```python
from build123d import *

# Parameters (mm, degrees)
SKETCH1_R               = 65
BULK_EXTRUDE_DEPTH      = 3
SKETCH2_R               = 40.5
SKETCH2_R_2             = 37.5
BEARING_RING_DEPTH      = 6
BEARING_START           = -1
SKETCH4_R               = 37.5
BEARING_CUT_DEPTH       = 1
SKETCH5_R               = 22
WIRE_PASSTHRU_CUT_DEPTH = 143.214667503


with BuildPart() as part:
    # Sketch1 → BULK EXTRUDE (new body)
    with BuildSketch(Plane(origin=(72, 0, 0), x_dir=(0, 0, -1), z_dir=(1, 0, 0))):
        with Locations((50, -18.372727273)):
            Circle(SKETCH1_R)
    extrude(amount=BULK_EXTRUDE_DEPTH)

    # Sketch2 → BEARING RING (add)
    with BuildSketch(Plane(origin=(75, 0, 0), x_dir=(0, 0, -1), z_dir=(1, 0, 0))):
        with Locations((50, -18.372727273)):
            Circle(SKETCH2_R)
        with Locations((50, -18.372727273)):
            Circle(SKETCH2_R_2, mode=Mode.SUBTRACT)
    extrude(amount=BEARING_RING_DEPTH)

    # Sketch4 → BEARING CUT (cut)
    with BuildSketch(Plane(origin=(75, 0, 0), x_dir=(0, 0, -1), z_dir=(1, 0, 0)).offset(BEARING_START)):
        with Locations((50, -18.372727273)):
            Circle(SKETCH4_R)
    extrude(amount=BEARING_CUT_DEPTH, mode=Mode.SUBTRACT)

    # Sketch5 → WIRE PASSTHRU CUT (cut, through all)
    with BuildSketch(Plane(origin=(74, 0, 0), x_dir=(0, 0, -1), z_dir=(1, 0, 0))):
        with Locations((50, -18.372727273)):
            Circle(SKETCH5_R)
    extrude(amount=-WIRE_PASSTHRU_CUT_DEPTH, mode=Mode.SUBTRACT)


solid = part.part
```
Geometry check sheet. Reference: the model listing, model coordinates, mm. A direction names the side the tool comes from. Give positions to 0.01 mm unless a question says otherwise; leave off trailing zeros. Loops run counter-clockwise (first coordinate to the right, second up) from the corner with the lowest first, then second, coordinate; pieces in that order, holes last. Notation, with made-up numbers: M 28.25,89 L 59.25,89 A35 ccw 59.25,128 Z; hole C 15.25,11.25 d10. An arc over 180 degrees is marked long. Write item = value, one per line.
(1) Sectioned sample at A-A, the plane z = -50. Record the cut outline in (x, y), plus the area to 3 significant figures.
Answer below:
outline = M 72,-83.37 L 75,-83.37 L 75,-58.87 L 81,-58.87 L 81,-55.87 L 74,-55.87 L 74,-40.37 L 72,-40.37 Z; M 72,3.63 L 74,3.63 L 74,19.13 L 81,19.13 L 81,22.13 L 75,22.13 L 75,46.63 L 72,46.63 Z
area = 263 mm2
(2) Sectioned sample at D-D, the plane y = -47. Record the cut outline in (x, z).
Answer below:
outline = M 72,-108.36 L 75,-108.36 L 75,-78.65 L 81,-78.65 L 81,-74.22 L 74,-74.22 L 74,-25.78 L 81,-25.78 L 81,-21.35 L 75,-21.35 L 75,8.36 L 72,8.36 Z
(3) Release check for a two-part mould opening along Z. For faces 3 (the face through (73.01, -26.8, -70.32)), 4 (the face through (75, 11.4, -78)), 5 (the face through (77.45, -7.11, -85.77)), 6 (the face through (77.958, -43.016, -17.861)) record: released by +Z, released by -Z, zero draft, split by the parting line, or undercut.
Answer below:
face_3 = undercut
face_4 = zero draft
face_5 = undercut
face_6 = split by the parting line
(4) Sectioned sample at C-C, the plane z = -75. Record the cut outline in (x, y).
Answer below:
outline = M 72,-78.37 L 75,-78.37 L 75,-50.24 L 81,-50.24 L 81,-46.32 L 74,-46.32 L 74,9.58 L 81,9.58 L 81,13.49 L 75,13.49 L 75,41.63 L 72,41.63 Z
(5) Sectioned sample at B-B, the plane y = -11.5. Record the cut outline in (x, z), plus the area to 3 significant figures.
Answer below:
outline = M 72,-114.64 L 75,-114.64 L 75,-89.91 L 81,-89.91 L 81,-86.86 L 74,-86.86 L 74,-70.9 L 72,-70.9 Z; M 72,-29.1 L 74,-29.1 L 74,-13.14 L 81,-13.14 L 81,-10.09 L 75,-10.09 L 75,14.64 L 72,14.64 Z
area = 267 mm2
(6) Material ranges on line 1 (Y direction, x = 73.1, z = -50); line 2 (Y direction, x = 77, z = -50); line 3 (Z direction, x = 77.75, y = -17), recorded low to high. Write a range as [from, to].
Answer below:
line_1 = [-83.37, -40.37], [3.63, 46.63]
line_2 = [-58.87, -55.87], [19.13, 22.13]
line_3 = [-90.48, -87.47], [-12.53, -9.52]
(7) Gauge pin test, flat ends, axial feed: pin 1 Ø5 at (x, y) = (79, -15) entering from -Z; pin 2 Ø3 at (y, z) = (23.5, -60.5) entering from +X; pin 3 Ø1 at (x, z) = (78, -69) entering from +Y. Record the tip position at first contact, or that the pin passes through.
Answer below:
pin_1 = -90.49
pin_2 = 75
pin_3 = 17.66
(8) Tool access check on faces 1 (the face through (74, -35, -66)), 2 (the face through (72, -17, -78)). Record the directions out of +Z, -Z, +X, -X, +Y, -Y that give a thin tool (end or side, any length) a straight path to the whole face; none if there is none.
Answer below:
face_1 = +X
face_2 = +Z, -Z, -X, +Y, -Y
